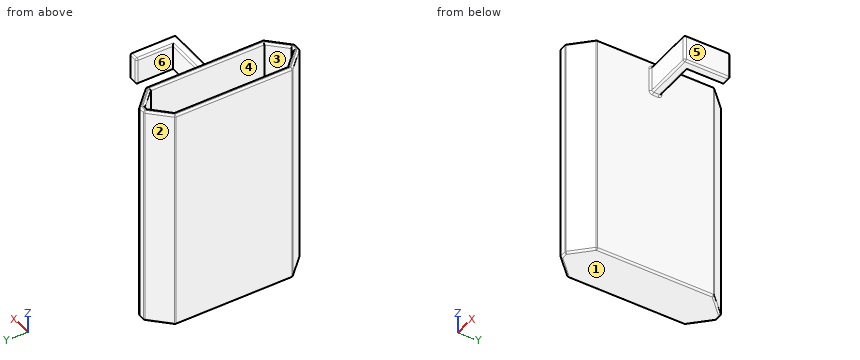
```python
from build123d import *

# Parameters (mm, degrees)
F1_DEPTH = 2.5
F2_DEPTH = 123.5
F3_W     = 5
F3_H     = 15
F4_DEPTH = 28.5
F5_START = 23
F3_W_2   = 20
F5_DEPTH = 5.5
F6_R     = 1


with BuildPart() as f1:
    # F0 (on Top) → F1 (new body)
    with BuildSketch(Plane.XY):
        Polygon((10, 31), (1, 40), (-1, 40), (-10, 31), (-10, -31), (-1, -40), (1, -40), (10, -31), align=None)
    extrude(amount=F1_DEPTH)

    # F0 (on Top) → F2 (join)
    with BuildSketch(Plane.XY):
        Polygon((12.500000447, -32.0355340911), (12.500000447, 32.0355340911), (2.0355340911, 42.500000447), (-2.0355340911, 42.500000447), (-12.500000447, 32.0355340911), (-12.500000447, -32.0355340911), (-2.0355340911, -42.500000447), (2.0355340911, -42.500000447), align=None)
        Polygon((-1, 40), (1, 40), (10, 31), (10, -31), (1, -40), (-1, -40), (-10, -31), (-10, 31), align=None, mode=Mode.SUBTRACT)
    extrude(amount=F2_DEPTH)

    # F3 (on face) → F4 (join)
    with BuildSketch(Plane.YZ.offset(12.500000447)):
        with Locations((-4.47e-07, 112.5)):
            Rectangle(F3_W, F3_H)
    extrude(amount=F4_DEPTH)

    # F3 (on face) → F5 (join)
    with BuildSketch(Plane.YZ.offset(12.500000447).offset(F5_START)):
        with Locations((12.499999553, 112.5)):
            Rectangle(F3_W_2, F3_H)
    extrude(amount=F5_DEPTH)

    # F6
    f6_edges = [f1.edges().sort_by_distance(p)[0] for p in [
        (12.5, 0, 123.5),
        (7.267767, 37.267767, 123.5),
        (0, 42.5, 123.5),
        (-7.267767, 37.267767, 123.5),
        (-12.5, 0, 123.5),
        (-7.267767, -37.267767, 123.5),
        (0, -42.5, 123.5),
        (7.267767, -37.267767, 123.5),
        (0, 40, 123.5),
        (5.5, 35.5, 123.5),
        (10, 0, 123.5),
        (5.5, -35.5, 123.5),
        (0, -40, 123.5),
        (-5.5, -35.5, 123.5),
        (-10, 0, 123.5),
        (-5.5, 35.5, 123.5),
        (24, 2.5, 120),
        (35.5, 12.5, 120),
        (38.25, 22.5, 120),
        (41, 10, 120),
        (26.75, -2.5, 120),
        (12.5, 0, 120),
        (26.75, -2.5, 105),
        (41, 10, 105),
        (38.25, 22.5, 105),
        (35.5, 12.5, 105),
        (24, 2.5, 105),
        (12.5, 0, 105),
        (12.5, 0, 0),
        (7.267767, 37.267767, 0),
        (0, 42.5, 0),
        (-7.267767, 37.267767, 0),
        (-12.5, 0, 0),
        (-7.267767, -37.267767, 0),
        (0, -42.5, 0),
        (7.267767, -37.267767, 0),
        (-2.035534, 42.5, 61.75),
        (-12.5, 32.035534, 61.75),
        (-12.5, -32.035534, 61.75),
        (-2.035534, -42.5, 61.75),
        (2.035534, 42.5, 61.75),
        (12.5, 32.035534, 61.75),
        (12.5, -32.035534, 61.75),
        (2.035534, -42.5, 61.75),
        (35.5, 22.5, 112.5),
        (41, 22.5, 112.5),
        (41, -2.5, 112.5),
        (12.5, 2.5, 112.5),
        (12.5, -2.5, 112.5),
    ]]
    fillet(f6_edges, radius=F6_R)


solid = f1.part
```
The listing builds one solid part. Answer for the finished solid, in the listing's coordinates (mm). Face numbers are marked on the shaded views. A direction names the side the tool comes from. Give positions to 0.01 mm unless a question says otherwise; leave off trailing zeros. Order: outer loops, then holes, each group sorted by start corner. A loop starts at its lowest first (then second) coordinate and runs counter-clockwise, first axis right, second up.
1) Consider line 1 along X through (y, z) = (15, 98.5); line 2 along X through (y, z) = (8, 110); line 3 along Y through (x, z) = (1, 19). Determine where each line is inside the solid, lowest interval first.
Reported:
line 1: x = -12.5 to -10, 10 to 12.5
line 2: x = -12.5 to -10, 10 to 12.5, 35.5 to 41
line 3: y = -42.5 to -40, 40 to 42.5
2) Find section A-A on y = 12. Write down the section's boundary in (x, z).
Reported:
outline: (-12.5, 1) arc R1 ccw to (-11.5, 0) - (11.5, 0) arc R1 ccw to (12.5, 1) - (12.5, 122.5) arc R1 ccw to (11.5, 123.5) - (11, 123.5) arc R1 ccw to (10, 122.5) - (10, 2.5) - (-10, 2.5) - (-10, 122.5) arc R1 ccw to (-11, 123.5) - (-11.5, 123.5) arc R1 ccw to (-12.5, 122.5) - close; (35.5, 106) arc R1 ccw to (36.5, 105) - (40, 105) arc R1 ccw to (41, 106) - (41, 119) arc R1 ccw to (40, 120) - (36.5, 120) arc R1 ccw to (35.5, 119) - close
3) Find section C-C on x = 32.5. Write down the section's boundary in (y, z), then the cut area to 3 significant figures.
Reported:
outline: (-2.5, 106) arc R1 ccw to (-1.5, 105) - (1.5, 105) arc R1 ccw to (2.5, 106) - (2.5, 119) arc R1 ccw to (1.5, 120) - (-1.5, 120) arc R1 ccw to (-2.5, 119) - close
area: 74.1 mm2
4) Given P1, Ø1.5, axis at x = -5, y = -6.5, coming from the +Z side; P2, Ø4, axis at x = -5, z = 35.5, coming from the -Y side; P3, Ø1, axis at x = 38.5, z = 111, coming from the +Y side, each flat-ended and moving along its own axis, determine where each tip first touches the part or whether it passes through.
Reported:
P1: stops at z = 2.5
P2: stops at y = -41.54
P3: stops at y = 22.5
5) Determine the mould class of the marked faces 1, 2, 3 and 4 for opening direction X: pulls with the +X half, pulls with the -X half, needs draft (parallel to the pull), parting line crosses it, or undercut.
Reported:
face 1: needs draft
face 2: pulls with the -X half
face 3: undercut
face 4: undercut
6) Find section B-B on z = 73.5. Write down the section's boundary in (x, y).
Reported:
outline: (-12.5, -31.62) arc R1 ccw to (-12.21, -32.33) - (-2.33, -42.21) arc R1 ccw to (-1.62, -42.5) - (1.62, -42.5) arc R1 ccw to (2.33, -42.21) - (12.21, -32.33) arc R1 ccw to (12.5, -31.62) - (12.5, 31.62) arc R1 ccw to (12.21, 32.33) - (2.33, 42.21) arc R1 ccw to (1.62, 42.5) - (-1.62, 42.5) arc R1 ccw to (-2.33, 42.21) - (-12.21, 32.33) arc R1 ccw to (-12.5, 31.62) - close; hole (-10, -31) - (-1, -40) - (1, -40) - (10, -31) - (10, 31) - (1, 40) - (-1, 40) - (-10, 31) - close
7) For the marked faces 5 and 6, determine the directions among +Z, -Z, +X, -X, +Y, -Y from which every point of the face is accessible in a straight line to the end or side of a thin tool.
Reported:
face 5: +Z, -Z, +X, +Y, -Y
face 6: +Z, -Z, +Y
